from build123d import *

# Parameters (mm, degrees)
F1_DEPTH = 3
F2_W     = 2.87808
F2_H     = 3
F2_W_2   = 0.06096
F3_DEPTH = 3.001


with BuildPart() as f1:
    # F0 (on Top) → F1 (new body)
    with BuildSketch(Plane.XY):
        with BuildLine():
            Line((0, 610.7938), (0, 814.4002))
            ThreePointArc((0, 814.4002), (-158.581862972, 798.8112909169), (-311.092710136, 752.6413564642))
            Line((-311.092710136, 752.6413564642), (-233.3171069657, 564.4751488911))
            ThreePointArc((-233.3171069657, 564.4751488911), (-222.21778397, 568.9361322731), (-211.0332265418, 573.1788930289))
            Line((-211.0332265418, 573.1788930289), (-211.0431366506, 573.2066473717))
            Line((-211.0431366506, 573.2066473717), (-205.3925469131, 575.2242760793))
            Line((-205.3925469131, 575.2242760793), (-199.7419556033, 577.2419053483))
            Line((-199.7419556033, 577.2419053483), (-199.7320454946, 577.2141510055))
            ThreePointArc((-199.7320454946, 577.2141510055), (-176.9750657056, 584.592928658), (-153.9465878827, 591.0748803643))
            Line((-153.9465878827, 591.0748803643), (-153.9537352346, 591.1034710825))
            Line((-153.9537352346, 591.1034710825), (-148.1328657869, 592.5586217348))
            Line((-148.1328657869, 592.5586217348), (-142.3119938407, 594.0137730116))
            Line((-142.3119938407, 594.0137730116), (-142.3048464889, 593.9851822935))
            ThreePointArc((-142.3048464889, 593.9851822935), (-118.9351607425, 599.1022397368), (-95.3830161725, 603.3002124517))
            Line((-95.3830161725, 603.3002124517), (-95.3873321972, 603.3293652515))
            Line((-95.3873321972, 603.3293652515), (-89.4520324924, 604.2080767429))
            Line((-89.4520324924, 604.2080767429), (-83.5167190162, 605.0867902733))
            Line((-83.5167190162, 605.0867902733), (-83.5124029915, 605.0576374735))
            ThreePointArc((-83.5124029915, 605.0576374735), (-59.7542154208, 607.8638826727), (-35.9043587106, 609.7376018781))
            Line((-35.9043587105, 609.7376018781), (-35.905802001, 609.7670370733))
            Line((-35.905802001, 609.7670370733), (-29.9129956796, 610.0608812306))
            Line((-29.9129956796, 610.0608812306), (-23.9202013429, 610.3547248004))
            Line((-23.9202013429, 610.3547248004), (-23.9187580524, 610.3252896052))
            ThreePointArc((-23.9187580524, 610.3252896052), (-11.9616730515, 610.6766611688), (0, 610.7938))
        make_face()
        with BuildLine():
            Line((-23.3325136158, 598.3691241423), (-23.9187580524, 610.3252896052))
            ThreePointArc((-23.9187580524, 610.3252896052), (-26.9162015413, 610.2004459299), (-29.9129956796, 610.0608812306))
            ThreePointArc((-29.9129956796, 610.0608812306), (-32.9090741607, 609.9065985512), (-35.9043587106, 609.7376018781))
            Line((-35.9043587105, 609.7376018781), (-35.3181142739, 597.7814364152))
            Line((-35.3181142739, 597.7814364152), (-23.3325136158, 598.3691241423))
        make_face()
        Polygon((-32.7015930533, 606.9205442942), (-26.830566427, 607.2084172504), (-26.6836444952, 604.2120170859), (-32.5546711216, 603.9241441296), align=None, mode=Mode.SUBTRACT)
        with BuildLine():
            ThreePointArc((-29.9129956796, 610.0608812306), (-26.9162015413, 610.2004459299), (-23.9187580524, 610.3252896052))
            Line((-23.9187580524, 610.3252896052), (-23.9202013429, 610.3547248004))
            Line((-23.9202013429, 610.3547248004), (-29.9129956796, 610.0608812306))
        make_face()
        with BuildLine():
            ThreePointArc((-35.9043587106, 609.7376018781), (-32.9090741607, 609.9065985512), (-29.9129956796, 610.0608812306))
            Line((-29.9129956796, 610.0608812306), (-35.905802001, 609.7670370733))
            Line((-35.905802001, 609.7670370733), (-35.9043587105, 609.7376018781))
        make_face()
        with BuildLine():
            Line((-211.0431366506, 573.2066473717), (-211.0332265418, 573.1788930289))
            ThreePointArc((-211.0332265418, 573.1788930289), (-208.2153983194, 574.2085109271), (-205.3925469131, 575.2242760793))
            Line((-205.3925469131, 575.2242760793), (-211.0431366506, 573.2066473717))
        make_face()
        with BuildLine():
            ThreePointArc((-205.3925469131, 575.2242760793), (-208.2153983194, 574.2085109271), (-211.0332265418, 573.1788930289))
            Line((-211.0332265418, 573.1788930289), (-207.0078786739, 561.9054663245))
            Line((-207.0078786739, 561.9054663245), (-195.7066976267, 565.9407243011))
            Line((-195.7066976267, 565.9407243011), (-199.7320454946, 577.2141510055))
            ThreePointArc((-199.7320454946, 577.2141510055), (-202.5647396363, 576.2261642572), (-205.3925469131, 575.2242760793))
        make_face()
        Polygon((-207.1516168949, 571.4106657146), (-201.6158463707, 573.3872964819), (-200.6070318766, 570.5620012201), (-206.1428024007, 568.5853704528), align=None, mode=Mode.SUBTRACT)
        with BuildLine():
            Line((-199.7419556033, 577.2419053483), (-205.3925469131, 575.2242760793))
            ThreePointArc((-205.3925469131, 575.2242760793), (-202.5647396363, 576.2261642572), (-199.7320454946, 577.2141510055))
            Line((-199.7320454946, 577.2141510055), (-199.7419556033, 577.2419053483))
        make_face()
        with BuildLine():
            Line((-81.7592939944, 593.2161770923), (-83.5124029915, 605.0576374735))
            ThreePointArc((-83.5124029915, 605.0576374735), (-86.4832609464, 604.6401505809), (-89.4520324924, 604.2080767429))
            ThreePointArc((-89.4520324924, 604.2080767429), (-92.4186391273, 603.7614274366), (-95.3830161725, 603.3002124517))
            Line((-95.3830161725, 603.3002124517), (-93.6299071754, 591.4587520705))
            Line((-93.6299071754, 591.4587520705), (-81.7592939944, 593.2161770923))
        make_face()
        Polygon((-91.9200199316, 600.8099959308), (-86.105318771, 601.6708530035), (-85.6659625155, 598.7031997082), (-91.4806636761, 597.8423426355), align=None, mode=Mode.SUBTRACT)
        with BuildLine():
            ThreePointArc((-89.4520324924, 604.2080767429), (-86.4832609464, 604.6401505809), (-83.5124029915, 605.0576374735))
            Line((-83.5124029915, 605.0576374735), (-83.5167190162, 605.0867902733))
            Line((-83.5167190162, 605.0867902733), (-89.4520324924, 604.2080767429))
        make_face()
        with BuildLine():
            ThreePointArc((-95.3830161725, 603.3002124517), (-92.4186391273, 603.7614274366), (-89.4520324924, 604.2080767429))
            Line((-89.4520324924, 604.2080767429), (-95.3873321972, 603.3293652515))
            Line((-95.3873321972, 603.3293652515), (-95.3830161725, 603.3002124517))
        make_face()
        with BuildLine():
            Line((-153.9537352346, 591.1034710825), (-153.9465878827, 591.0748803643))
            ThreePointArc((-153.9465878827, 591.0748803643), (-151.0415487687, 591.8238899064), (-148.1328657869, 592.5586217348))
            Line((-148.1328657869, 592.5586217348), (-153.9537352346, 591.1034710825))
        make_face()
        with BuildLine():
            ThreePointArc((-148.1328657869, 592.5586217348), (-151.0415487687, 591.8238899064), (-153.9465878827, 591.0748803643))
            Line((-153.9465878827, 591.0748803643), (-151.0434333054, 579.4617296886))
            Line((-151.0434333054, 579.4617296886), (-139.4016919116, 582.3720316178))
            Line((-139.4016919116, 582.3720316178), (-142.3048464889, 593.9851822935))
            ThreePointArc((-142.3048464889, 593.9851822935), (-145.2206078584, 593.2790584301), (-148.1328657869, 592.5586217348))
        make_face()
        Polygon((-150.2565843576, 588.9353955501), (-144.5539937532, 590.3609778471), (-143.8264182709, 587.4505424986), (-149.5290088753, 586.0249602016), align=None, mode=Mode.SUBTRACT)
        with BuildLine():
            Line((-142.3119938407, 594.0137730116), (-148.1328657869, 592.5586217348))
            ThreePointArc((-148.1328657869, 592.5586217348), (-145.2206078584, 593.2790584301), (-142.3048464889, 593.9851822935))
            Line((-142.3048464889, 593.9851822935), (-142.3119938407, 594.0137730116))
        make_face()
    extrude(amount=F1_DEPTH)

    # F2 (on face) → F3 (cut, through all)
    with BuildSketch(Plane.XY.offset(3)):
        with Locations((-4.5, 636.2446)):
            Rectangle(F2_W, F2_H)
        with Locations((-4.5, 687.1462)):
            Rectangle(F2_W, F2_H)
        with Locations((-4.5, 738.0478)):
            Rectangle(F2_W, F2_H)
        with Locations((-4.5, 788.9494)):
            Rectangle(F2_W, F2_H)
        with Locations((4.5, 687.1462)):
            Rectangle(F2_W, F2_H)
        with Locations((3.03048, 687.1462)):
            Rectangle(F2_W_2, F2_H)
        with Locations((5.96952, 687.1462)):
            Rectangle(F2_W_2, F2_H)
        with Locations((3.03048, 788.9494)):
            Rectangle(F2_W_2, F2_H)
        with Locations((4.5, 788.9494)):
            Rectangle(F2_W, F2_H)
        with Locations((5.96952, 788.9494)):
            Rectangle(F2_W_2, F2_H)
        with Locations((3.03048, 636.2446)):
            Rectangle(F2_W_2, F2_H)
        with Locations((4.5, 636.2446)):
            Rectangle(F2_W, F2_H)
        with Locations((5.96952, 636.2446)):
            Rectangle(F2_W_2, F2_H)
        with Locations((3.03048, 738.0478)):
            Rectangle(F2_W_2, F2_H)
        with Locations((4.5, 738.0478)):
            Rectangle(F2_W, F2_H)
        with Locations((5.96952, 738.0478)):
            Rectangle(F2_W_2, F2_H)
        Polygon((-260.2834437092, 637.5696963512), (-259.1374737912, 634.7971969468), (-259.0811366033, 634.8204830556), (-260.2271065213, 637.5929824599), align=None)
        Polygon((-260.2271065213, 637.5929824599), (-259.0811366033, 634.8204830556), (-256.4213115748, 635.9198807561), (-257.5672814928, 638.6923801604), align=None)
        Polygon((-257.5672814928, 638.6923801604), (-256.4213115748, 635.9198807561), (-256.3649743869, 635.9431668648), (-257.5109443049, 638.7156662692), align=None)
        Polygon((-278.5250373959, 681.8620349488), (-279.6710073139, 684.6345343532), (-279.7273445018, 684.6112482444), (-278.5813745838, 681.8387488401), align=None)
        Polygon((-277.0111822853, 685.7339320537), (-279.6710073139, 684.6345343532), (-278.5250373959, 681.8620349488), (-275.8652123674, 682.9614326494), align=None)
        Polygon((-276.9548450974, 685.7572181624), (-277.0111822853, 685.7339320537), (-275.8652123674, 682.9614326494), (-275.8088751795, 682.9847187581), align=None)
        Polygon((-299.1712452944, 731.6528001377), (-298.0252753764, 728.8803007334), (-297.9689381885, 728.9035868421), (-299.1149081065, 731.6760862465), align=None)
        Polygon((-299.1149081065, 731.6760862465), (-297.9689381885, 728.9035868421), (-295.3091131599, 730.0029845426), (-296.4550830779, 732.775483947), align=None)
        Polygon((-296.4550830779, 732.775483947), (-295.3091131599, 730.0029845426), (-295.252775972, 730.0262706514), (-296.39874589, 732.7987700557), align=None)
        Polygon((-239.6935729986, 587.7556450535), (-239.6372358107, 587.7789311623), (-240.7832057287, 590.5514305666), (-240.8395429166, 590.5281444579), align=None)
        Polygon((-240.7832057287, 590.5514305666), (-239.6372358107, 587.7789311623), (-236.9774107822, 588.8783288628), (-238.1233807002, 591.6508282671), align=None)
        Polygon((-238.1233807002, 591.6508282671), (-236.9774107822, 588.8783288628), (-236.9210735943, 588.9016149715), (-238.0670435123, 591.6741143759), align=None)
    extrude(amount=-F3_DEPTH, mode=Mode.SUBTRACT)


solid = f1.part
The model under review builds one solid part; all positions refer to its coordinate system, in mm. A direction names the side the tool comes from. Give positions to 0.01 mm unless a question says otherwise; leave off trailing zeros. Order: outer loops, then holes, each group sorted by start corner. A loop starts at its lowest first (then second) coordinate and runs counter-clockwise, first axis right, second up. Notation, with made-up numbers: M 29.5,59.5 L 64.5,59.5 A31 ccw 64.5,88.5 Z; hole C -15.5,59 d7. An arc over 180 degrees is marked long. Answer in a Markdown table with one row per item. Add a question column.
1. For pin 1 Ø0.9 at (y, z) = (738, 1) entering from -X; pin 2 Ø1.5 at (y, z) = (687.5, 1) entering from -X, all flat-tipped, find the tip position at first contact; note any pin that passes through.
2. Add section C-C on y = 780.5. State the section outline as (x, z) points.
3. To check wall thickness, follow line 1 along Y through (x, z) = (-256.5, 2.7); line 2 along X through (y, z) = (732.5, 1.55); line 3 along Y through (x, z) = (-239, 1.05). State the ranges of each line that lie inside material, in increasing order.
4. Add section A-A on z = 2.3. Count the separate pieces of the cut face and the enclosed holes in it, plus the area to 3 significant figures.
5. Machinability: for faces 1 (the flat face through (-272.75, 659.88, 1.48)), 2 (the cylindrical face through (-222.374, 568.875, 1.479)), which of the approach directions +Z, -Z, +X, -X, +Y, -Y give a long, thin tool a straight path to every point of the face, cutting with its end or side? Answer none if there is none.
6. Add section B-B on x = -122.5. State the section outline as (y, z) points, plus the area to 3 significant figures.
7. Mouldability with a two-part tool opening along X and no side actions: class faces 3 (the flat face through (-158, 690, 3)), 4 (the cylindrical face through (-119.264, 599.037, 1.479)), 5 (the cylindrical face through (-156.39, 799.243, 1.479)), 6 (the cylindrical face through (-177.296, 584.496, 1.479)) as released by +X, released by -X, zero draft, split by the parting line, or undercut.
The answers:
| question | item | result |
|---|---|---|
| 1 | pin 1 | x = -305.23 |
| 1 | pin 2 | x = -284.48 |
| 2 | outline | M -232.52,0 L 0,0 L 0,3 L -232.52,3 Z |
| 3 | line 1 | 620.56 to 635.89, 636.27 to 772.95 |
| 3 | line 2 | -302.77 to -297.12, -296.28 to 0 |
| 3 | line 3 | 578.22 to 588.04, 591.29 to 778.54 |
| 4 | separate pieces | 1 |
| 4 | enclosed holes | 12 |
| 4 | area | 57,300 mm2 |
| 5 | face 1 | +Z, -Z, -X, -Y |
| 5 | face 2 | +Z, -Z, -Y |
| 6 | outline | M 598.38,0 L 805.13,0 L 805.13,3 L 598.38,3 Z |
| 6 | area | 620 mm2 |
| 7 | face 3 | zero draft |
| 7 | face 4 | undercut |
| 7 | face 5 | released by -X |
| 7 | face 6 | undercut |
